Autodesk Inventor part; units mm, degrees
ref_plane "YZ Plane" through (0, 0, 0) normal (1, 0, 0) x (0, 1, 0)
ref_plane "XZ Plane" through (0, 0, 0) normal (0, 1, 0) x (-1, 0, 0)
ref_plane "XY Plane" through (0, 0, 0) normal (0, 0, 1) x (1, 0, 0)
sketch "Sketch1" plane through (0, 0, 0) normal (0, 0, 1) x (1, 0, 0)
  circle A0 centre (0, 0) radius 7
  circle A1 centre (0, 0) radius 5.75
  circle A2 centre (0, 0) radius 4.25
  dimension "d0" = 14
  dimension "d1" = 11.5
  dimension "d6" = 8.5
extrude "Extrusion1" add sketch "Sketch1" along normal blind 8 contours A1 | A2
extrude "Extrusion2" add sketch "Sketch1" against normal blind 1.5 contours A0 | A1 | A2
extrude "Extrusion3" cut sketch "Sketch1" along normal up to next contours A2
properties part number "Rodend12mil"
Part model, mm, in its own coordinate system. A direction names the side the tool comes from. Give positions to 0.01 mm unless a question says otherwise; leave off trailing zeros. Order: outer loops, then holes, each group sorted by start corner. A loop starts at its lowest first (then second) coordinate and runs counter-clockwise, first axis right, second up. Notation, with made-up numbers: (25, 8) - (74, 8) arc R14 ccw to (74, 16) - close; hole circle Ø11 at (89.5, 73). An arc over 180 degrees is marked (long way). Use a Markdown table: item, result.
1) Two-plate mould, pull along X, no slides. Class faces 1 (the flat face through (-1, 6, 0)), 2 (the cylindrical face through (6.466, -2.681, -0.74)), 3 (the cylindrical face through (2.285, -3.584, 3.944)), 4 (the flat face through (0, 0, 0)): +X half, -X half, draft (parallel to the pull), parting line (faces both ways), or undercut.
Checked values:
| item | result |
|---|---|
| face 1 | draft |
| face 2 | parting line |
| face 3 | undercut |
| face 4 | undercut |
2) Flat gauge pins, fed straight in: P1, Ø5, axis at x = 0, z = 1, coming from the +Y side; P2, Ø3, axis at x = -4.5, z = 3.5, coming from the -Y side; P3, Ø3, axis at x = 2.5, z = 1, coming from the +Y side; P4, Ø3, axis at x = -5, z = 2.5, coming from the +Y side. Where does each tip first touch, or does it go through?
Checked values:
| item | result |
|---|---|
| P1 | y = 7 |
| P2 | y = -4.91 |
| P3 | y = 6.86 |
| P4 | y = 4.56 |
3) Saw through at C-C on z = 1.25. List the corners of the cut face in (x, y), plus the area to 3 significant figures.
Checked values:
| item | result |
|---|---|
| outline | circle Ø11.5 at (0, 0); hole circle Ø8.5 at (0, 0) |
| area | 47.1 mm² |
4) Probe L1, parallel to Y at x = 0, z = 3; L2, parallel to Z at x = -2.5, y = 1.75; L3, parallel to X at y = 0.5, z = 6.5. List the from-to ranges inside material, lowest first. Write a range as from..to.
Checked values:
| item | result |
|---|---|
| L1 | -5.75..-4.25, 4.25..5.75 |
| L2 | -1.5..0 |
| L3 | -5.73..-4.22, 4.22..5.73 |
5) 3-axis set-ups, long thin cutter, end or side, ignore diameter. For faces 5 (the flat face through (0, 0, -1.5)), 6 (the cylindrical face through (-0.75, -5.7, 3.94)): which of +Z, -Z, +X, -X, +Y, -Y reach the whole face in a straight line?
Checked values:
| item | result |
|---|---|
| face 5 | -Z, +X, -X, +Y, -Y |
| face 6 | +Z |
6) Saw through at D-D on z = -0.5. List the corners of the cut face in (x, y).
Checked values:
| item | result |
|---|---|
| outline | circle Ø14 at (0, 0) |
7) Saw through at A-A on x = 0. List the corners of the cut face in (y, z).
Checked values:
| item | result |
|---|---|
| outline | (-7, -1.5) - (7, -1.5) - (7, 0) - (5.75, 0) - (5.75, 8) - (4.25, 8) - (4.25, 0) - (-4.25, 0) - (-4.25, 8) - (-5.75, 8) - (-5.75, 0) - (-7, 0) - close |
